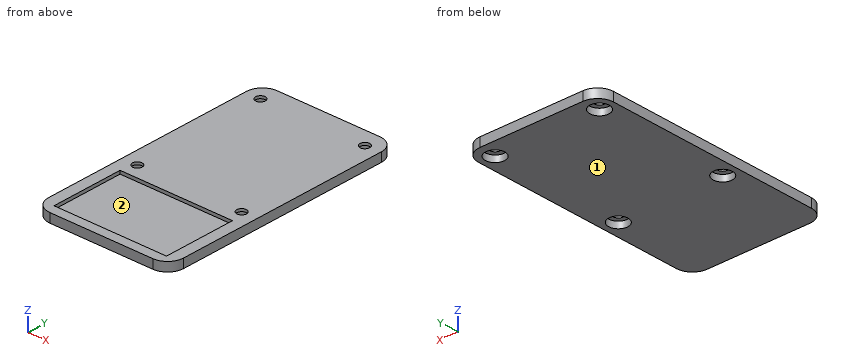
from build123d import *

# Parameters (mm, degrees)
F0_R     = 3
F0_R_2   = 1.5
F1_DEPTH = 2.8
F2_DEPTH = 2
F3_W     = 35
F3_H     = 22.5
F4_DEPTH = 1


with BuildPart() as f1:
    # F0 (on Top) → F1 (new body)
    with BuildSketch(Plane.XY):
        with BuildLine():
            Line((16, 38.7), (-16, 38.7))
            ThreePointArc((-16, 38.7), (-19.535534, 37.235534), (-21, 33.7))
            Line((-21, 33.7), (-21, -33.7))
            ThreePointArc((-21, -33.7), (-19.535534, -37.235534), (-16, -38.7))
            Line((-16, -38.7), (16, -38.7))
            ThreePointArc((16, -38.7), (19.535534, -37.235534), (21, -33.7))
            Line((21, -33.7), (21, 33.7))
            ThreePointArc((21, 33.7), (19.535534, 37.235534), (16, 38.7))
        make_face()
        with Locations((-16.25, -8.7)):
            Circle(F0_R, mode=Mode.SUBTRACT)
        with BuildLine():
            ThreePointArc((19.25, -8.7), (16.25, -11.7), (13.25, -8.7))
            ThreePointArc((13.25, -8.7), (16.25, -5.7), (19.25, -8.7))
        make_face(mode=Mode.SUBTRACT)
        with Locations((-16.25, 33.3)):
            Circle(F0_R, mode=Mode.SUBTRACT)
        with BuildLine():
            ThreePointArc((19.25, 33.3), (16.25, 30.3), (13.25, 33.3))
            ThreePointArc((13.25, 33.3), (16.25, 36.3), (19.25, 33.3))
        make_face(mode=Mode.SUBTRACT)
        with Locations((-16.25, 33.3)):
            Circle(F0_R)
        with Locations((-16.25, 33.3)):
            Circle(F0_R_2, mode=Mode.SUBTRACT)
        with BuildLine():
            ThreePointArc((19.25, 33.3), (16.25, 36.3), (13.25, 33.3))
            ThreePointArc((13.25, 33.3), (16.25, 30.3), (19.25, 33.3))
        make_face()
        with BuildLine():
            ThreePointArc((17.75, 33.3), (16.25, 31.8), (14.75, 33.3))
            ThreePointArc((14.75, 33.3), (16.25, 34.8), (17.75, 33.3))
        make_face(mode=Mode.SUBTRACT)
        with Locations((-16.25, -8.7)):
            Circle(F0_R)
        with Locations((-16.25, -8.7)):
            Circle(F0_R_2, mode=Mode.SUBTRACT)
        with BuildLine():
            ThreePointArc((19.25, -8.7), (16.25, -5.7), (13.25, -8.7))
            ThreePointArc((13.25, -8.7), (16.25, -11.7), (19.25, -8.7))
        make_face()
        with BuildLine():
            ThreePointArc((17.75, -8.7), (16.25, -10.2), (14.75, -8.7))
            ThreePointArc((14.75, -8.7), (16.25, -7.2), (17.75, -8.7))
        make_face(mode=Mode.SUBTRACT)
    extrude(amount=F1_DEPTH)

    # F0 (on Top) → F2 (cut)
    with BuildSketch(Plane.XY):
        with BuildLine():
            ThreePointArc((19.25, 33.3), (16.25, 36.3), (13.25, 33.3))
            ThreePointArc((13.25, 33.3), (16.25, 30.3), (19.25, 33.3))
        make_face()
        with BuildLine():
            ThreePointArc((17.75, 33.3), (16.25, 31.8), (14.75, 33.3))
            ThreePointArc((14.75, 33.3), (16.25, 34.8), (17.75, 33.3))
        make_face(mode=Mode.SUBTRACT)
        with Locations((-16.25, 33.3)):
            Circle(F0_R)
        with Locations((-16.25, 33.3)):
            Circle(F0_R_2, mode=Mode.SUBTRACT)
        with BuildLine():
            ThreePointArc((19.25, -8.7), (16.25, -5.7), (13.25, -8.7))
            ThreePointArc((13.25, -8.7), (16.25, -11.7), (19.25, -8.7))
        make_face()
        with BuildLine():
            ThreePointArc((17.75, -8.7), (16.25, -10.2), (14.75, -8.7))
            ThreePointArc((14.75, -8.7), (16.25, -7.2), (17.75, -8.7))
        make_face(mode=Mode.SUBTRACT)
        with Locations((-16.25, -8.7)):
            Circle(F0_R)
        with Locations((-16.25, -8.7)):
            Circle(F0_R_2, mode=Mode.SUBTRACT)
    extrude(amount=F2_DEPTH, mode=Mode.SUBTRACT)

    # F3 (on face) → F4 (cut)
    with BuildSketch(Plane.XY.offset(2.8)):
        with Locations((0, -24.45)):
            Rectangle(F3_W, F3_H)
    extrude(amount=-F4_DEPTH, mode=Mode.SUBTRACT)


solid = f1.part
Model file for the job. Use its own axes, mm. Face numbers are marked on the shaded views. Give positions to 0.01 mm unless a question says otherwise; leave off trailing zeros. Order: outer loops, then holes, each group sorted by start corner. A loop starts at its lowest first (then second) coordinate and runs counter-clockwise, first axis right, second up. Notation, with made-up numbers: (25.5, -20.5) - (35.5, -20.5) arc R22 ccw to (35.5, 16.5) - close; hole circle Ø2 at (15.5, -28.5). An arc over 180 degrees is marked (long way). Write item = value, one per line. Start each with the question number.
1. Drop flat-ended pins along their axis: P1, Ø5.5, axis at x = -16.25, y = 33.3, coming from the -Z side; P2, Ø1.8, axis at x = -16.25, y = -8.7, coming from the -Z side. Give the stop position or say it passes through.
2. Cut at A-A, the plane y = -8.7. List the corners of the cut face in (x, z).
3. Cut at D-D, the plane y = -24. List the corners of the cut face in (x, z).
4. Cut at B-B, the plane x = -2.5. List the corners of the cut face in (y, z), and give its area (3 significant figures).
5. Two-plate mould, pull along Y, no slides. Class the marked faces 1 and 2: pulls with the +Y half, pulls with the -Y half, needs draft (parallel to the pull), parting line crosses it, or undercut.
6. Probe line 1 along Y through (x, z) = (16.25, 2.2); line 2 along Y through (x, z) = (16.25, 0.6); line 3 along X through (y, z) = (-22.5, 2.3). List the from-to ranges inside material, lowest first.
7. Cut at C-C, the plane z = 0.7. List the corners of the cut face in (x, y), and give its area (3 significant figures).
Taken from the geometry:
q1.P1 = 2
q1.P2 = through
q2.outline = (-21, 0) - (-19.25, 0) - (-19.25, 2) - (-17.75, 2) - (-17.75, 2.8) - (-21, 2.8) - close; (-14.75, 2) - (-13.25, 2) - (-13.25, 0) - (13.25, 0) - (13.25, 2) - (14.75, 2) - (14.75, 2.8) - (-14.75, 2.8) - close; (17.75, 2) - (19.25, 2) - (19.25, 0) - (21, 0) - (21, 2.8) - (17.75, 2.8) - close
q3.outline = (-21, 0) - (21, 0) - (21, 2.8) - (17.5, 2.8) - (17.5, 1.8) - (-17.5, 1.8) - (-17.5, 2.8) - (-21, 2.8) - close
q4.outline = (-38.7, 0) - (38.7, 0) - (38.7, 2.8) - (-13.2, 2.8) - (-13.2, 1.8) - (-35.7, 1.8) - (-35.7, 2.8) - (-38.7, 2.8) - close
q4.area = 194 mm²
q5.face_1 = needs draft
q5.face_2 = undercut
q6.line_1 = -38.69 to -35.7, -13.2 to -10.2, -7.2 to 31.8, 34.8 to 38.69
q6.line_2 = -38.69 to -11.7, -5.7 to 30.3, 36.3 to 38.69
q6.line_3 = -21 to -17.5, 17.5 to 21
q7.outline = (-21, -33.7) arc R5 ccw to (-16, -38.7) - (16, -38.7) arc R5 ccw to (21, -33.7) - (21, 33.7) arc R5 ccw to (16, 38.7) - (-16, 38.7) arc R5 ccw to (-21, 33.7) - close; hole circle Ø6 at (-16.25, -8.7); hole circle Ø6 at (-16.25, 33.3); hole circle Ø6 at (16.25, -8.7); hole circle Ø6 at (16.25, 33.3)
q7.area = 3,120 mm²
